Here's how the part is built. I have some questions about the finished solid (model axes, mm). Face numbers are marked on the shaded views. A direction names the side the tool comes from. Round coordinates to 2 decimals unless told otherwise and drop trailing zeros. Loops run counter-clockwise (first coordinate to the right, second up) from the corner with the lowest first, then second, coordinate; pieces in that order, holes last. Notation, with made-up numbers: M 87,13 L 106,13 A15 cw 106,18 Z; hole C -12.5,-0.75 d8. An arc over 180 degrees is marked long. Answer as a JSON object with one key per item and string values.
from build123d import *

# Parameters (mm, degrees)
F0_R     = 62.5
F1_DEPTH = 50
F3_DEPTH = 15
F4_R     = 11
F5_DEPTH = 50.001
F7_DEPTH = 50.001
F8_SIZE  = 3


with BuildPart() as f1:
    # F0 (on Top) → F1 (new body)
    with BuildSketch(Plane.XY):
        Circle(F0_R)
    extrude(amount=F1_DEPTH)

    # F2 (on face) → F3 (join)
    with BuildSketch(Plane.XY.offset(50)):
        with BuildLine():
            ThreePointArc((-8.5, 26.153394), (0, 27.5), (8.5, 26.153394))
            Line((8.5, 26.153394), (13.136364, 40.418881))
            ThreePointArc((13.136364, 40.418881), (0, 42.5), (-13.136364, 40.418881))
            Line((-13.136364, 40.418881), (-8.5, 26.153394))
        make_face()
        with BuildLine():
            Line((-39.791143, 14.930338), (-25.74721, 9.660807))
            ThreePointArc((-25.74721, 9.660807), (-21.500366, 17.14597), (-15.147883, 22.951942))
            Line((-15.147883, 22.951942), (-23.410365, 35.471183))
            ThreePointArc((-23.410365, 35.471183), (-33.227838, 26.498317), (-39.791143, 14.930338))
        make_face()
        with BuildLine():
            Line((-36.482379, -21.801055), (-23.606246, -14.106565))
            ThreePointArc((-23.606246, -14.106565), (-26.810518, -6.119326), (-27.389101, 2.46721))
            Line((-27.389101, 2.46721), (-42.328611, 3.81296))
            ThreePointArc((-42.328611, 3.81296), (-41.434436, -9.45714), (-36.482379, -21.801055))
        make_face()
        with BuildLine():
            Line((-5.701641, -42.115808), (-3.689297, -27.251405))
            ThreePointArc((-3.689297, -27.251405), (-11.931803, -24.776644), (-19.005768, -19.875382))
            Line((-19.005768, -19.875382), (-29.37255, -30.716499))
            ThreePointArc((-29.37255, -30.716499), (-18.440059, -38.291177), (-5.701641, -42.115808))
        make_face()
        with BuildLine():
            Line((29.37255, -30.716499), (19.005768, -19.875382))
            ThreePointArc((19.005768, -19.875382), (11.931803, -24.776644), (3.689297, -27.251405))
            Line((3.689297, -27.251405), (5.701641, -42.115808))
            ThreePointArc((5.701641, -42.115808), (18.440059, -38.291177), (29.37255, -30.716499))
        make_face()
        with BuildLine():
            Line((42.328611, 3.81296), (27.389101, 2.46721))
            ThreePointArc((27.389101, 2.46721), (26.810518, -6.119326), (23.606246, -14.106565))
            Line((23.606246, -14.106565), (36.482379, -21.801055))
            ThreePointArc((36.482379, -21.801055), (41.434436, -9.45714), (42.328611, 3.81296))
        make_face()
        with BuildLine():
            Line((23.410365, 35.471183), (15.147883, 22.951942))
            ThreePointArc((15.147883, 22.951942), (21.500366, 17.14597), (25.74721, 9.660807))
            Line((25.74721, 9.660807), (39.791143, 14.930338))
            ThreePointArc((39.791143, 14.930338), (33.227838, 26.498317), (23.410365, 35.471183))
        make_face()
    extrude(amount=F3_DEPTH)

    # F4 (on face) → F5 (cut, through all)
    with BuildSketch(Plane.XY.offset(50)):
        Circle(F4_R)
    extrude(amount=-F5_DEPTH, mode=Mode.SUBTRACT)

    # F6 (on face) → F7 (cut, through all)
    with BuildSketch(Plane.XY.offset(50)):
        with BuildLine():
            ThreePointArc((-40.466334, 26.25), (-41.077894, 28.646163), (-42.762973, 30.456167))
            ThreePointArc((-42.762973, 30.456167), (-44.164755, 28.385285), (-45.466334, 26.25))
            ThreePointArc((-45.466334, 26.25), (-46.664755, 24.055158), (-47.757301, 21.805738))
            ThreePointArc((-47.757301, 21.805738), (-42.863915, 21.980642), (-40.466334, 26.25))
        make_face()
        with BuildLine():
            ThreePointArc((-45.466334, 26.25), (-44.164755, 28.385285), (-42.762973, 30.456167))
            ThreePointArc((-42.762973, 30.456167), (-49.796461, 28.75), (-47.757301, 21.805738))
            ThreePointArc((-47.757301, 21.805738), (-46.664755, 24.055158), (-45.466334, 26.25))
        make_face()
        with BuildLine():
            ThreePointArc((4.994328, 52.261905), (4.998582, 52.380919), (5, 52.5))
            ThreePointArc((5, 52.5), (-0.119081, 57.498582), (-4.994328, 52.261905))
            ThreePointArc((-4.994328, 52.261905), (0, 52.5), (4.994328, 52.261905))
        make_face()
        with BuildLine():
            ThreePointArc((4.994328, 52.261905), (0, 52.5), (-4.994328, 52.261905))
            ThreePointArc((-4.994328, 52.261905), (0, 47.5), (4.994328, 52.261905))
        make_face()
        with BuildLine():
            ThreePointArc((-42.762973, -30.456167), (-41.077894, -28.646163), (-40.466334, -26.25))
            ThreePointArc((-40.466334, -26.25), (-42.863915, -21.980642), (-47.757301, -21.805738))
            ThreePointArc((-47.757301, -21.805738), (-46.664755, -24.055158), (-45.466334, -26.25))
            ThreePointArc((-45.466334, -26.25), (-44.164755, -28.385285), (-42.762973, -30.456167))
        make_face()
        with BuildLine():
            ThreePointArc((-45.466334, -26.25), (-46.664755, -24.055158), (-47.757301, -21.805738))
            ThreePointArc((-47.757301, -21.805738), (-49.796461, -28.75), (-42.762973, -30.456167))
            ThreePointArc((-42.762973, -30.456167), (-44.164755, -28.385285), (-45.466334, -26.25))
        make_face()
        with BuildLine():
            ThreePointArc((-4.994328, -52.261905), (-0.119081, -57.498582), (5, -52.5))
            ThreePointArc((5, -52.5), (4.998582, -52.380919), (4.994328, -52.261905))
            ThreePointArc((4.994328, -52.261905), (2.5, -52.440442), (0, -52.5))
            ThreePointArc((0, -52.5), (-2.5, -52.440442), (-4.994328, -52.261905))
        make_face()
        with BuildLine():
            ThreePointArc((0, -52.5), (2.5, -52.440442), (4.994328, -52.261905))
            ThreePointArc((4.994328, -52.261905), (0, -47.5), (-4.994328, -52.261905))
            ThreePointArc((-4.994328, -52.261905), (-2.5, -52.440442), (0, -52.5))
        make_face()
        with BuildLine():
            ThreePointArc((42.762973, -30.456167), (47.862497, -30.638439), (50.466334, -26.25))
            ThreePointArc((50.466334, -26.25), (49.735692, -23.647582), (47.757301, -21.805738))
            ThreePointArc((47.757301, -21.805738), (45.466334, -26.25), (42.762973, -30.456167))
        make_face()
        with BuildLine():
            ThreePointArc((42.762973, -30.456167), (45.466334, -26.25), (47.757301, -21.805738))
            ThreePointArc((47.757301, -21.805738), (41.136207, -23.75), (42.762973, -30.456167))
        make_face()
        with BuildLine():
            ThreePointArc((47.757301, 21.805738), (49.735692, 23.647582), (50.466334, 26.25))
            ThreePointArc((50.466334, 26.25), (47.862497, 30.638439), (42.762973, 30.456167))
            ThreePointArc((42.762973, 30.456167), (44.164755, 28.385285), (45.466334, 26.25))
            ThreePointArc((45.466334, 26.25), (46.664755, 24.055158), (47.757301, 21.805738))
        make_face()
        with BuildLine():
            ThreePointArc((45.466334, 26.25), (44.164755, 28.385285), (42.762973, 30.456167))
            ThreePointArc((42.762973, 30.456167), (41.136207, 23.75), (47.757301, 21.805738))
            ThreePointArc((47.757301, 21.805738), (46.664755, 24.055158), (45.466334, 26.25))
        make_face()
    extrude(amount=-F7_DEPTH, mode=Mode.SUBTRACT)

    # F8
    f8_edges = [f1.edges().sort_by_distance(p)[0] for p in [
        (-62.5, 0, 50),
        (-62.5, 0, 0),
    ]]
    chamfer(f8_edges, length=F8_SIZE)


solid = f1.part
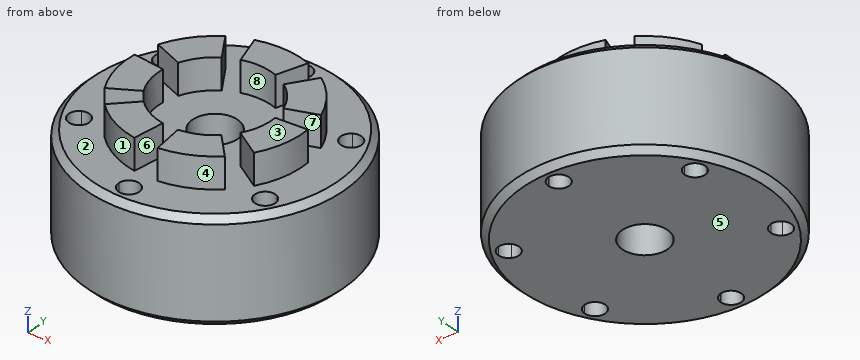
Item 1: If I drill on L1, parallel to Y at x = 45, z = 16.5; L2, parallel to Y at x = -44, z = 5; L3, parallel to X at y = 0.5, z = 57.5, over which ranges is the centre line in solid material (lowest first)? Write a range as from..to.
Solution:
{"L1": "y = -43.37..-31.23, -21.27..21.27, 31.23..43.37", "L2": "y = -44.39..-31.03, -21.47..21.47, 31.03..44.39", "L3": "x = -42.5..-27.5, 27.5..42.5"}
Item 2: For the marked faces 1, 2, 3 and 4, which set-ups out of +Z, -Z, +X, -X, +Y, -Y let a thin tool reach every point of the face, with its end or its side?
Solution:
{"face 1": "+Z, -X, -Y", "face 2": "+Z", "face 3": "+Z, +X, -X, +Y, -Y", "face 4": "+Z, +X, -Y"}
Item 3: I want a section at C-C on z = 25. List the corners of the cut face in (x, y) for me, plus the area to 3 significant figures.
Solution:
{"outline": "C 0,0 d125; hole M -47.76,-21.81 A5 ccw long -42.76,-30.46 A5 ccw -40.47,-26.25 A5 ccw Z; hole M -47.76,21.81 A5 ccw -40.47,26.25 A5 ccw -42.76,30.46 A5 ccw long Z; hole C 0,0 d22; hole M 4.99,-52.26 A5 ccw long 5,-52.5 A5 ccw Z; hole M 4.99,52.26 A5 ccw 5,52.5 A5 ccw long Z; hole M 42.76,-30.46 A5 ccw 50.47,-26.25 A5 ccw long Z; hole M 42.76,30.46 A5 ccw long 50.47,26.25 A5 ccw Z", "area": "11,400 mm2"}
Item 4: For P1, Ø2, axis at y = 12, z = 45.5, coming from the +X side; P2, Ø4, axis at y = -12, z = 10.5, coming from the +X side; P3, Ø5, axis at x = -8, z = 37.5, coming from the +Y side, each with a flat end and sliding along its axis, tell me the tip position at first contact or that it passes through.
Solution:
{"P1": "stops at x = 61.52", "P2": "stops at x = 61.69", "P3": "stops at y = 62.26"}
Item 5: I want a section at A-A on x = 0. List the corners of the cut face in (y, z) for me.
Solution:
{"outline": "M -62.5,3 L -59.5,0 L -57.5,0 L -57.5,50 L -59.5,50 L -62.5,47 Z; M -47.5,0 L -11,0 L -11,50 L -47.5,50 Z; M 11,0 L 47.5,0 L 47.5,50 L 42.5,50 L 42.5,65 L 27.5,65 L 27.5,50 L 11,50 Z; M 57.5,0 L 59.5,0 L 62.5,3 L 62.5,47 L 59.5,50 L 57.5,50 Z"}
Item 6: We'd pull the mould along Y, two halves only. Please class the marked faces 5, 6, 7 and 8: +Y half, -Y half, draft (parallel to the pull), parting line (faces both ways), or undercut.
Solution:
{"face 5": "draft", "face 6": "-Y half", "face 7": "undercut", "face 8": "undercut"}
Item 7: I want a section at B-B on y = 0. List the corners of the cut face in (x, z) for me, plus the area to 3 significant figures.
Solution:
{"outline": "M -62.5,3 L -59.5,0 L -11,0 L -11,50 L -27.5,50 L -27.5,65 L -42.5,65 L -42.5,50 L -59.5,50 L -62.5,47 Z; M 11,0 L 59.5,0 L 62.5,3 L 62.5,47 L 59.5,50 L 42.5,50 L 42.5,65 L 27.5,65 L 27.5,50 L 11,50 Z", "area": "5,580 mm2"}
